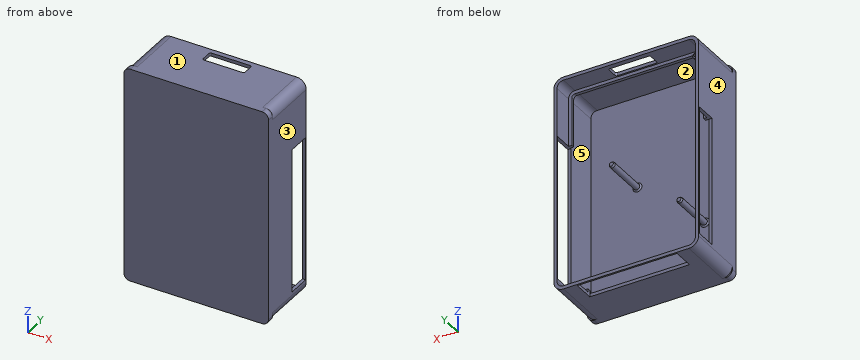
```python
from build123d import *
from OCP.BRepFilletAPI import BRepFilletAPI_MakeChamfer

# Parameters (mm, degrees)
EXTRUDE_1_DEPTH     = 2
EXTRUDE_2_DEPTH     = 17.5
SKETCH_3_R          = 0.9
EXTRUDE_3_DEPTH     = 13.5
CHAMFER_2_SIZE      = 0.5
CHAMFER_2_SIZE2     = 0.288675135
CHAMFER_3_SIZE      = 0.5
CHAMFER_3_SIZE2     = 0.288675135
CHAMFER_4_SIZE      = 0.5
CHAMFER_4_SIZE2     = 0.288675135
EXTRUDE_5_DEPTH     = 1
CUT_EXTRUDE_1_REACH = 75.318
CUT_EXTRUDE_2_REACH = 61.393
SKETCH_7_W          = 45
SKETCH_7_H          = 7
CUT_EXTRUDE_3_REACH = 61.393
CUT_EXTRUDE_4_REACH = 75.318
SKETCH_9_W          = 31
SKETCH_9_H          = 6.5


with BuildPart() as part:
    # 草图1 → 凸台-拉伸1 (new body)
    with BuildSketch(Plane(origin=(0, 0, 0), x_dir=(1, 0, 0), z_dir=(0, 1, 0))):
        with BuildLine():
            Line((-22.5, 31.5), (-22.5, -31.5))
            ThreePointArc((-22.5, -31.5), (-21.914213562, -32.914213562), (-20.5, -33.5))
            Line((-20.5, -33.5), (20.5, -33.5))
            ThreePointArc((20.5, -33.5), (21.914213562, -32.914213562), (22.5, -31.5))
            Line((22.5, -31.5), (22.5, 31.5))
            ThreePointArc((22.5, 31.5), (21.914213562, 32.914213562), (20.5, 33.5))
            Line((20.5, 33.5), (-20.5, 33.5))
            ThreePointArc((-20.5, 33.5), (-21.914213562, 32.914213562), (-22.5, 31.5))
        make_face()
    extrude(amount=EXTRUDE_1_DEPTH)

    # 草图2 → 凸台-拉伸2 (add)
    with BuildSketch(Plane(origin=(0, 2, 0), x_dir=(1, 0, 0), z_dir=(0, 1, 0))):
        with BuildLine():
            Line((19.5, 33.5), (-19.5, 33.5))
            ThreePointArc((-19.5, 33.5), (-21.621320344, 32.621320344), (-22.5, 30.5))
            Line((-22.5, 30.5), (-22.5, -30.5))
            ThreePointArc((-22.5, -30.5), (-21.621320344, -32.621320344), (-19.5, -33.5))
            Line((-19.5, -33.5), (19.5, -33.5))
            ThreePointArc((19.5, -33.5), (21.621320344, -32.621320344), (22.5, -30.5))
            Line((22.5, -30.5), (22.5, 30.5))
            ThreePointArc((22.5, 30.5), (21.621320344, 32.621320344), (19.5, 33.5))
        make_face()
        with BuildLine():
            Line((-21.5, 30.5), (-21.5, -30.5))
            ThreePointArc((-21.5, -30.5), (-20.914213562, -31.914213562), (-19.5, -32.5))
            Line((-19.5, -32.5), (19.5, -32.5))
            ThreePointArc((19.5, -32.5), (20.914213562, -31.914213562), (21.5, -30.5))
            Line((21.5, -30.5), (21.5, 30.5))
            ThreePointArc((21.5, 30.5), (20.914213562, 31.914213562), (19.5, 32.5))
            Line((19.5, 32.5), (-19.5, 32.5))
            ThreePointArc((-19.5, 32.5), (-20.914213562, 31.914213562), (-21.5, 30.5))
        make_face(mode=Mode.SUBTRACT)
    extrude(amount=EXTRUDE_2_DEPTH)

    # 草图3 → 凸台-拉伸3 (add)
    with BuildSketch(Plane(origin=(0, 2, 0), x_dir=(1, 0, 0), z_dir=(0, 1, 0))):
        with Locations(Location((-14, 14, 0), (0, 0, 90))):
            Circle(SKETCH_3_R)
        with Locations(Location((7, -4, 0), (0, 0, 90))):
            Circle(SKETCH_3_R)
        with Locations(Location((-19, -30, 0), (0, 0, 90))):
            Circle(SKETCH_3_R)
    extrude(amount=EXTRUDE_3_DEPTH)

    # 倒角2: one chamfer whose edges measure the first distance from different faces: ONE call of the kernel's chamfer builder (chamfer() names one face for all edges)
    chamfer_2_edges_1 = [part.edges().sort_by_distance(p)[0] for p in [
        (-14, 2, -13.1),
    ]]
    chamfer_2_side_1 = [part.faces().sort_by_distance(p)[0] for p in [
        (0.023765643, 2, -0.018281264),
    ]]
    chamfer_2_edges_2 = [part.edges().sort_by_distance(p)[0] for p in [
        (-14, 15.5, -13.1),
    ]]
    chamfer_2_side_2 = [part.faces().sort_by_distance(p)[0] for p in [
        (-14, 8.75, -13.1),
    ]]
    chamfer_2 = BRepFilletAPI_MakeChamfer(part.part.solid().wrapped)
    for e in chamfer_2_edges_1:
        chamfer_2.Add(CHAMFER_2_SIZE, CHAMFER_2_SIZE2, e.wrapped, chamfer_2_side_1[0].wrapped)  # the first distance lies on this face
    for e in chamfer_2_edges_2:
        chamfer_2.Add(CHAMFER_2_SIZE, CHAMFER_2_SIZE2, e.wrapped, chamfer_2_side_2[0].wrapped)  # the first distance lies on this face
    add(Compound.cast(chamfer_2.Shape()), mode=Mode.REPLACE)

    # 倒角3: one chamfer whose edges measure the first distance from different faces: ONE call of the kernel's chamfer builder (chamfer() names one face for all edges)
    chamfer_3_edges_1 = [part.edges().sort_by_distance(p)[0] for p in [
        (7, 2, 4.9),
    ]]
    chamfer_3_side_1 = [part.faces().sort_by_distance(p)[0] for p in [
        (0.04198855, 2, -0.000112994),
    ]]
    chamfer_3_edges_2 = [part.edges().sort_by_distance(p)[0] for p in [
        (7, 15.5, 4.9),
    ]]
    chamfer_3_side_2 = [part.faces().sort_by_distance(p)[0] for p in [
        (7, 8.75, 4.9),
    ]]
    chamfer_3 = BRepFilletAPI_MakeChamfer(part.part.solid().wrapped)
    for e in chamfer_3_edges_1:
        chamfer_3.Add(CHAMFER_3_SIZE, CHAMFER_3_SIZE2, e.wrapped, chamfer_3_side_1[0].wrapped)  # the first distance lies on this face
    for e in chamfer_3_edges_2:
        chamfer_3.Add(CHAMFER_3_SIZE, CHAMFER_3_SIZE2, e.wrapped, chamfer_3_side_2[0].wrapped)  # the first distance lies on this face
    add(Compound.cast(chamfer_3.Shape()), mode=Mode.REPLACE)

    # 倒角4: one chamfer whose edges measure the first distance from different faces: ONE call of the kernel's chamfer builder (chamfer() names one face for all edges)
    chamfer_4_edges_1 = [part.edges().sort_by_distance(p)[0] for p in [
        (-19, 2, 30.9),
    ]]
    chamfer_4_side_1 = [part.faces().sort_by_distance(p)[0] for p in [
        (-19, 8.75, 30.9),
    ]]
    chamfer_4_edges_2 = [part.edges().sort_by_distance(p)[0] for p in [
        (-19, 15.5, 30.9),
    ]]
    chamfer_4_side_2 = [part.faces().sort_by_distance(p)[0] for p in [
        (-19, 15.5, 30),
    ]]
    chamfer_4 = BRepFilletAPI_MakeChamfer(part.part.solid().wrapped)
    for e in chamfer_4_edges_1:
        chamfer_4.Add(CHAMFER_4_SIZE, CHAMFER_4_SIZE2, e.wrapped, chamfer_4_side_1[0].wrapped)  # the first distance lies on this face
    for e in chamfer_4_edges_2:
        chamfer_4.Add(CHAMFER_4_SIZE, CHAMFER_4_SIZE2, e.wrapped, chamfer_4_side_2[0].wrapped)  # the first distance lies on this face
    add(Compound.cast(chamfer_4.Shape()), mode=Mode.REPLACE)

    # 草图6 → 凸台-拉伸5 (add)
    with BuildSketch(Plane(origin=(0, 12.5, 0), x_dir=(1, 0, 0), z_dir=(0, 1, 0))):
        with BuildLine():
            Line((-21.5, 30.5), (-21.5, -30.5))
            ThreePointArc((-21.5, -30.5), (-20.914213562, -31.914213562), (-19.5, -32.5))
            Line((-19.5, -32.5), (19.5, -32.5))
            ThreePointArc((19.5, -32.5), (20.914213562, -31.914213562), (21.5, -30.5))
            Line((21.5, -30.5), (21.5, 30.5))
            ThreePointArc((21.5, 30.5), (20.914213562, 31.914213562), (19.5, 32.5))
            Line((19.5, 32.5), (-19.5, 32.5))
            ThreePointArc((-19.5, 32.5), (-20.914213562, 31.914213562), (-21.5, 30.5))
        make_face()
        with BuildLine():
            Line((19.5, 31.5), (-19.5, 31.5))
            ThreePointArc((-19.5, 31.5), (-20.207106781, 31.207106781), (-20.5, 30.5))
            Line((-20.5, 30.5), (-20.5, -30.5))
            ThreePointArc((-20.5, -30.5), (-20.207106781, -31.207106781), (-19.5, -31.5))
            Line((-19.5, -31.5), (19.5, -31.5))
            ThreePointArc((19.5, -31.5), (20.207106781, -31.207106781), (20.5, -30.5))
            Line((20.5, -30.5), (20.5, 30.5))
            ThreePointArc((20.5, 30.5), (20.207106781, 31.207106781), (19.5, 31.5))
        make_face(mode=Mode.SUBTRACT)
    extrude(amount=EXTRUDE_5_DEPTH)

    # 草图4 → 切除-拉伸1 (cut, up to next)
    with BuildSketch(Plane.XY.offset(33.5), mode=Mode.PRIVATE) as cut_extrude_1_sk1:
        with BuildLine():
            Line((-6.5, 17.5), (-6.5, 14.5))
            ThreePointArc((-6.5, 14.5), (-6.353553391, 14.146446609), (-6, 14))
            Line((-6, 14), (6, 14))
            ThreePointArc((6, 14), (6.353553391, 14.146446609), (6.5, 14.5))
            Line((6.5, 14.5), (6.5, 17.5))
            ThreePointArc((6.5, 17.5), (6.353553391, 17.853553391), (6, 18))
            Line((6, 18), (-6, 18))
            ThreePointArc((-6, 18), (-6.353553391, 17.853553391), (-6.5, 17.5))
        make_face()
    cut_extrude_1_tool1 = extrude(cut_extrude_1_sk1.sketch, amount=-CUT_EXTRUDE_1_REACH, mode=Mode.PRIVATE) & part.part
    add(cut_extrude_1_tool1.solids().sort_by_distance((0, 16, 33.5))[0], mode=Mode.SUBTRACT)

    # 草图7 → 切除-拉伸2 (cut, up to next)
    with BuildSketch(Plane(origin=(22.5, 0, 0), x_dir=(0, 0, -1), z_dir=(1, 0, 0)), mode=Mode.PRIVATE) as cut_extrude_2_sk1:
        with Locations((7, 15.73884151)):
            Rectangle(SKETCH_7_W, SKETCH_7_H)
    cut_extrude_2_tool1 = extrude(cut_extrude_2_sk1.sketch, amount=-CUT_EXTRUDE_2_REACH, mode=Mode.PRIVATE) & part.part
    add(cut_extrude_2_tool1.solids().sort_by_distance((22.5, 15.738842, -7))[0], mode=Mode.SUBTRACT)

    # 草图8 → 切除-拉伸3 (cut, up to next)
    with BuildSketch(Plane.ZY.offset(22.5), mode=Mode.PRIVATE) as cut_extrude_3_sk1:
        Polygon((-29.5, 19), (-29.5, 12.5), (10.5, 12.5), (10.5, 15.014135881), (10.5, 19), align=None)
    cut_extrude_3_tool1 = extrude(cut_extrude_3_sk1.sketch, amount=-CUT_EXTRUDE_3_REACH, mode=Mode.PRIVATE) & part.part
    add(cut_extrude_3_tool1.solids().sort_by_distance((-22.5, 15.75, -9.5))[0], mode=Mode.SUBTRACT)

    # 草图9 → 切除-拉伸4 (cut, up to next)
    with BuildSketch(Plane(origin=(0, 0, -33.5), x_dir=(-1, 0, 0), z_dir=(0, 0, -1)), mode=Mode.PRIVATE) as cut_extrude_4_sk1:
        with Locations((0, 15.75)):
            Rectangle(SKETCH_9_W, SKETCH_9_H)
    cut_extrude_4_tool1 = extrude(cut_extrude_4_sk1.sketch, amount=-CUT_EXTRUDE_4_REACH, mode=Mode.PRIVATE) & part.part
    add(cut_extrude_4_tool1.solids().sort_by_distance((0, 15.75, -33.5))[0], mode=Mode.SUBTRACT)


solid = part.part
```
Build history of the part. All positions in model axes, mm. Face numbers are marked on the shaded views. A direction names the side the tool comes from. Coordinates: 2 decimals unless noted, no trailing zeros. Order: outer loops, then holes, each group sorted by start corner. A loop starts at its lowest first (then second) coordinate and runs counter-clockwise, first axis right, second up. Notation, with made-up numbers: (53.25, 23.5) -> (60.25, 23.5) arc R21 cw to (60.25, 59.5) -> close; hole circle Ø9 at (74.5, 35.25). An arc over 180 degrees is marked (long way). Answer in a Markdown table with one row per item. Add a question column.
Q1. Band-saw the part on C-C, the plane z = -19. List the corners of the cut face in (x, y).
Q2. Which spindle directions (+Z, -Z, +X, -X, +Y, -Y) get a long thin tool onto all of the face, cutting with end or side? Do the marked faces 4 and 5. Say none if no direction does.
Q3. Band-saw the part on D-D, the plane z = 22. List the corners of the cut face in (x, y), then the cut area to 3 significant figures.
Q4. Drop flat-ended pins along their axis: pin 1 (0.5 mm diameter, centred on y = 15.5, z = 33, fed in from +X); pin 2 (0.5 mm diameter, centred on x = -22, z = -10, fed in from -Y); pin 3 (2 mm diameter, centred on y = 17, z = -32, fed in from +X); pin 4 (0.8 mm diameter, centred on y = 16.5, z = 33, fed in from -X). Give the stop position or say it passes through.
Q5. Band-saw the part on A-A, the plane y = 10. List the corners of the cut face in (x, z), then the cut area to 3 significant figures.
Q6. Wall check: line 1 along X through (y, z) = (10, 4); line 2 along X through (y, z) = (8, 2.5); line 3 along Z through (x, y) = (-7.5, 11.25). Give the ranges that are in metal, low to high. Write a range as [from, to].
Q7. Mould opens along Z. For the marked faces 1, 2 and 3 say: +Z half, -Z half, draft (parallel to the pull), parting line (faces both ways), or undercut.
Q8. Band-saw the part on B-B, the plane x = -10.5. List the corners of the cut face in (y, z), then the cut area to 4 significant figures.
Answers follow:
| question | item | result |
|---|---|---|
| 1 | outline | (-22.5, 0) -> (22.5, 0) -> (22.5, 12.24) -> (21.5, 12.24) -> (21.5, 2) -> (-21.5, 2) -> (-21.5, 12.5) -> (-22.5, 12.5) -> close; (-22.5, 19) -> (-21.5, 19) -> (-21.5, 19.5) -> (-22.5, 19.5) -> close; (21.5, 19.24) -> (22.5, 19.24) -> (22.5, 19.5) -> (21.5, 19.5) -> close |
| 2 | face 4 | +Z, -Z, -X, +Y, -Y |
| 2 | face 5 | none |
| 3 | outline | (-22.5, 0) -> (22.5, 0) -> (22.5, 19.5) -> (21.5, 19.5) -> (21.5, 13.5) -> (20.5, 13.5) -> (20.5, 12.5) -> (21.5, 12.5) -> (21.5, 2) -> (-21.5, 2) -> (-21.5, 12.5) -> (-20.5, 12.5) -> (-20.5, 13.5) -> (-21.5, 13.5) -> (-21.5, 19.5) -> (-22.5, 19.5) -> close |
| 3 | area | 127 mm^2 |
| 4 | pin 1 | x = 21.48 |
| 4 | pin 2 | y = 0 |
| 4 | pin 3 | x = 22.46 |
| 4 | pin 4 | x = -21.64 |
| 5 | outline | (-22.5, -30.5) arc R3 ccw to (-19.5, -33.5) -> (19.5, -33.5) arc R3 ccw to (22.5, -30.5) -> (22.5, 30.5) arc R3 ccw to (19.5, 33.5) -> (-19.5, 33.5) arc R3 ccw to (-22.5, 30.5) -> close; circle Ø1.8 at (-19, 30); circle Ø1.8 at (-14, -14); circle Ø1.8 at (7, 4); hole (-21.5, -30.5) arc R2 ccw to (-19.5, -32.5) -> (19.5, -32.5) arc R2 ccw to (21.5, -30.5) -> (21.5, 30.5) arc R2 ccw to (19.5, 32.5) -> (-19.5, 32.5) arc R2 ccw to (-21.5, 30.5) -> close |
| 5 | area | 223 mm^2 |
| 6 | line 1 | [-22.5, -21.5], [6.1, 7.9], [21.5, 22.5] |
| 6 | line 2 | [-22.5, -21.5], [21.5, 22.5] |
| 6 | line 3 | [-33.5, -32.5], [32.5, 33.5] |
| 7 | face 1 | +Z half |
| 7 | face 2 | undercut |
| 7 | face 3 | draft |
| 8 | outline | (0, -33.5) -> (12.5, -33.5) -> (12.5, -32.5) -> (2, -32.5) -> (2, 32.5) -> (12.5, 32.5) -> (12.5, 31.5) -> (13.5, 31.5) -> (13.5, 32.5) -> (19.5, 32.5) -> (19.5, 33.5) -> (0, 33.5) -> close; (19, -33.5) -> (19.5, -33.5) -> (19.5, -32.5) -> (19, -32.5) -> close |
| 8 | area | 163.5 mm^2 |
